Verification items for the finished model (mm, model axes). A direction names the side the tool comes from. Coordinates: 2 decimals unless noted, no trailing zeros. Loops run counter-clockwise (first coordinate to the right, second up) from the corner with the lowest first, then second, coordinate; pieces in that order, holes last.
Q1. Sectioned sample at B-B (y = 1). Enter the section's corners in (x, z).
Q2. Go/stop test with flat-tipped pins: P1, Ø2, axis at x = 2.5, z = 9, coming from the -Y side; P2, Ø5, axis at y = -11, z = 8, coming from the -X side; P3, Ø4.5, axis at y = -34, z = 2.5, coming from the -X side; P4, Ø8.5, axis at x = 2, y = -65, coming from the +Z side. Record where each tip stops, or that it passes through.
Q3. Sectioned sample at D-D (z = 13). Enter the section's corners in (x, y), then the cut area to 3 significant figures.
Q4. Material ranges on probe 1 along Y at (x, z) = (0, 1); probe 2 along Y at (x, z) = (0, 7.5); probe 3 along Z at (x, y) = (11, -59), recorded low to high.
Q5. Sectioned sample at A-A (x = 0). Enter the section's corners in (y, z), then the cut area to 3 significant figures.
Q6. Sectioned sample at C-C (y = -20). Enter the section's corners in (x, z), then the cut area to 3 significant figures.
Q7. Mould release check, pull along X, two halves, no side actions. Record for faces 6 (the face through (0, 3, 2)), 7 (the face through (11, -22, 2)), 8 (the face through (0, -20, 3.9)), 9 (the face through (0, -58, 3.9)): +X half, -X half, draft (parallel to the pull), parting line (faces both ways), or undercut.
Q8. Access from +Z, -Z, +X, -X, +Y, -Y to the whole of each face (thin tool, end or side, straight path). Record for faces 1 (the face through (9, -22, 3.9)), 2 (the face through (7.795, -45.694, 8.83)), 3 (the face through (0.715, -0.375, 1.923)), 4 (the face through (-9, -22, 3.9)), 5 (the face through (-11, -22, 2)).
```python
from build123d import *

# Parameters (mm, degrees)
SKETCH_R      = 1.55
PAD_DEPTH     = 3.9
PAD002_DEPTH  = 47
SKETCH001_R   = 15.5
SKETCH001_R_2 = 14.5
PAD003_DEPTH  = 10


with BuildPart() as part:
    # Sketch → Pad (new body)
    with BuildSketch(Plane.XY):
        with BuildLine():
            Line((-11, 3), (11, 3))
            Line((11, 3), (11, -47))
            ThreePointArc((-11, -47), (0, -73.420165), (11, -47))
            Line((-11, 3), (-11, -47))
        make_face()
        with Locations((0, 1)):
            Circle(SKETCH_R, mode=Mode.SUBTRACT)
    extrude(amount=PAD_DEPTH)

    # Sketch003 (on Face1 of Pad) → Pad002 (join)
    with BuildSketch(Plane(origin=(0, 3, 0), x_dir=(-1, 0, 0), z_dir=(0, 1, 0))):
        with BuildLine():
            ThreePointArc((-6, 3.9), (-6.5, 4.4), (-7, 3.9))
            Line((-7, 3.9), (-6, 3.9))
        make_face()
        with BuildLine():
            ThreePointArc((7, 3.9), (6.5, 4.4), (6, 3.9))
            Line((6, 3.9), (7, 3.9))
        make_face()
    extrude(amount=-PAD002_DEPTH)

    # Sketch001 (on Face5 of Pad002) → Pad003 (join)
    with BuildSketch(Plane.XY.offset(3.9)):
        with Locations((0, -57.920165)):
            Circle(SKETCH001_R)
        with Locations((0, -57.920165)):
            Circle(SKETCH001_R_2, mode=Mode.SUBTRACT)
    extrude(amount=PAD003_DEPTH)


solid = part.part
```
Geometry check:
1. outline: (-11, 0) - (-1.55, 0) - (-1.55, 3.9) - (-6, 3.9) arc R0.5 ccw to (-7, 3.9) - (-11, 3.9) - close; (1.55, 0) - (11, 0) - (11, 3.9) - (7, 3.9) arc R0.5 ccw to (6, 3.9) - (1.55, 3.9) - close
2. P1: stops at y = -73.35
2. P2: passes through
2. P3: stops at x = -11
2. P4: stops at z = 3.9
3. outline: circle Ø31 at (0, -57.92); hole circle Ø29 at (0, -57.92)
3. area: 94.2 mm2
4. probe 1: y = -73.42 to -0.55, 2.55 to 3
4. probe 2: y = -73.42 to -72.42, -43.42 to -42.42
4. probe 3: z = 0 to 3.9
5. outline: (-73.42, 0) - (-0.55, 0) - (-0.55, 3.9) - (-42.42, 3.9) - (-42.42, 13.9) - (-43.42, 13.9) - (-43.42, 3.9) - (-72.42, 3.9) - (-72.42, 13.9) - (-73.42, 13.9) - close; (2.55, 0) - (3, 0) - (3, 3.9) - (2.55, 3.9) - close
5. area: 306 mm2
6. outline: (-11, 0) - (11, 0) - (11, 3.9) - (7, 3.9) arc R0.5 ccw to (6, 3.9) - (-6, 3.9) arc R0.5 ccw to (-7, 3.9) - (-11, 3.9) - close
6. area: 86.6 mm2
7. face 6: draft
7. face 7: +X half
7. face 8: undercut
7. face 9: undercut
8. face 1: +Z, +X, +Y
8. face 2: +Z
8. face 3: +Z, -Z
8. face 4: +Z, -X, +Y
8. face 5: +Z, -Z, -X, +Y
